Autodesk Inventor part; units mm, degrees
ref_plane "YZ Plane" through (0, 0, 0) normal (1, 0, 0) x (0, 1, 0)
ref_plane "XY Plane" through (0, 0, 0) normal (0, 0, 1) x (1, 0, 0)
sketch "Sketch1" plane through (0, 0, 0) normal (0, 0, 1) x (1, 0, 0)
  circle A0 centre (0, 0) radius 50
  circle A1 centre (0, 0) radius 40
  dimension "d0" = 100
  dimension "d1" = 80
extrude "Extrusion1" add sketch "Sketch1" against normal blind 500
ref_plane "Work Plane1" through (0, 0, -500) normal (0, 0, -1) x (-1, 0, 0)
sketch "Sketch2" plane through (0, 0, -500) normal (0, 0, -1) x (-1, 0, 0)
  circle A0 centre (0, 0) radius 50
  circle A1 centre (0, 0) radius 40
  line L0 (0, 0) -> (0, 50)
sketch "Sketch3" plane through (0, 0, 0) normal (0, 1, 0) x (-1, 0, 0)
  point P0 (0, 0)
sketch "Sketch4" plane through (0, 0, 0) normal (0, 1, 0) x (-1, 0, 0)
  line L0 (70, -500) -> (-70, -500)
  line L1 (-50, -500) -> (50, -500)
  circle A0 centre (0, -500) radius 40
  circle A1 centre (0, -500) radius 50
  point P0 (0, 0)
  point P1 (40, -500)
  point P2 (-40, -500)
  dimension "d5" = 80
  dimension "d6" = 100
sketch "Sketch6" plane through (0, 0, 0) normal (0, 1, 0) x (-1, 0, 0)
  point P0 (0, 0)
sketch "Sketch7" plane through (0, 0, 0) normal (0, 1, 0) x (-1, 0, 0)
  line L0 (-40, -500) -> (-40, -500)
  circle A0 centre (0, -500) radius 40
  line L1 (-50, -500) -> (-50, -500)
  circle A1 centre (0, -500) radius 50
  point P0 (0, 0)
  point P1 (50, -400)
  point P2 (40, -400)
ref_plane "Work Plane4" through (50, 0, -500) normal (0, 0.7071, -0.7071) x (-1, 0, 0)
split "Split2" plane through (50, 0, -500) removes the side toward (0, 0.7071, -0.7071)
extrude "Extrusion3" add sketch "Sketch7" along normal blind 680
revolve "Revolution2" add sketch "Sketch4" angle 90 about axis through (0, 0, -500) along (-1, 0, 0) picked at (-46.3464, -503.2515) contours A1 L0 A0
ref_plane "Work Plane5" through (0, 680, -500) normal (0, 1, 0) x (1, 0, 0)
properties part number "Z3" material "Steel, Alloy"
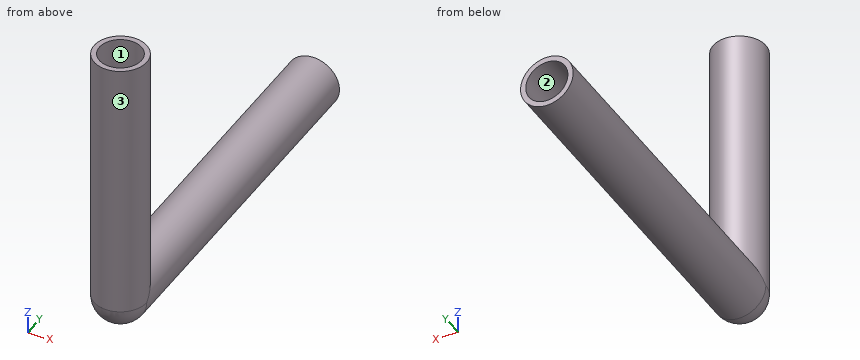
Work out the finished part from the listing and answer in its coordinate system (mm). Face numbers are marked on the shaded views. Give positions to 0.01 mm unless a question says otherwise; leave off trailing zeros. Order: outer loops, then holes, each group sorted by start corner. A loop starts at its lowest first (then second) coordinate and runs counter-clockwise, first axis right, second up. Notation, with made-up numbers: M 30.5,-37 L 78.5,-37 A20 ccw 78.5,-26 Z; hole C -6,18 d9. An arc over 180 degrees is marked long. Return JSON: item names as keys, results as strings.
Q1. Find section A-A, the plane x = 0. Write down the section's boundary in (y, z).
Answer below:
{"outline": "M -50,-500 A50 ccw 0,-550 L 680,-550 L 680,-540 L 0,-540 A40 cw -40,-500 L -40,0 L -50,0 Z; M 0,-460 L 680,-460 L 680,-450 L 50,-450 L 50,0 L 40,0 L 40,-450 L 0,-450 Z"}
Q2. The mould has two halves that part along X. Classify the marked faces 1, 2 and 3: pulls with the +X half, pulls with the -X half, needs draft (parallel to the pull), parting line crosses it, or undercut.
Answer below:
{"face 1": "undercut", "face 2": "undercut", "face 3": "parting line crosses it"}
Q3. Find section C-C, the plane z = -413.5. Write down the section's boundary in (x, y).
Answer below:
{"outline": "C 0,0 d100; hole C 0,0 d80"}
Q4. Find section B-B, the plane y = 245.5. Write down the section's boundary in (x, z).
Answer below:
{"outline": "C 0,-500 d100; hole C 0,-500 d80"}
Q5. Each of these flat-tipped pins is pushed along its axis until it touches: pin 1 (8 mm diameter, centred on x = 31, y = 101, fed in from +Z); pin 2 (12 mm diameter, centred on x = -17, z = -98.5, fed in from -Y) (3 decimals); pin 3 (10 mm diameter, centred on x = -10.5, z = -117, fed in from -Y). Where does it stop, or does it pass through?
Answer below:
{"pin 1": "stops at z = -457.92", "pin 2": "stops at y = -48.775", "pin 3": "stops at y = -49.7"}
Q6. Find section D-D, the plane x = -32.5. Write down the section's boundary in (y, z), and give its area (3 significant figures).
Answer below:
{"outline": "M -38,-500 A38 ccw 0,-538 L 680,-538 L 680,-523.32 L 0,-523.32 A23.32 cw -23.32,-500 L -23.32,0 L -38,0 Z; M 0,-476.68 L 680,-476.68 L 680,-462 L 38,-462 L 38,0 L 23.32,0 L 23.32,-462 L 0,-462 Z", "area": "34,800 mm^2"}
Q7. Find the intervals of material crossed by line 1 along Z through (x, y) = (0, 231); line 2 along Y through (x, z) = (0, -151), in increasing order. Write a range as [from, to].
Answer below:
{"line 1": "z = [-550, -540], [-460, -450]", "line 2": "y = [-50, -40], [40, 50]"}
